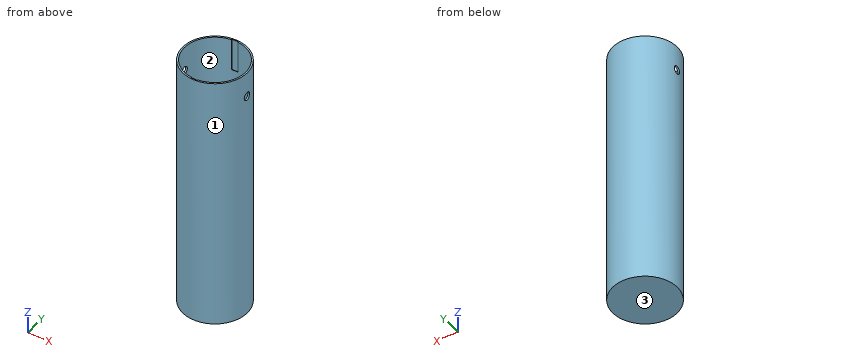
from build123d import *

# Parameters (mm, degrees)
SKETCH1_R           = 10
BOSS_EXTRUDE1_DEPTH = 80
SHELL1_T            = -0.5
SKETCH4_R           = 1.25
CUT_EXTRUDE3_DEPTH  = 84.066238629
SKETCH8_W           = 2
SKETCH8_H           = 0.25
CUT_EXTRUDE5_DEPTH  = 10


with BuildPart() as part:
    # Sketch1 → Boss-Extrude1 (new body)
    with BuildSketch(Plane.XY):
        Circle(SKETCH1_R)
    extrude(amount=BOSS_EXTRUDE1_DEPTH)

    # Shell1
    shell1_openings = [part.faces().sort_by_distance(p)[0] for p in [
        (0, 0, 80),
    ]]
    offset(amount=SHELL1_T, openings=shell1_openings, kind=Kind.INTERSECTION)

    # Sketch4 → Cut-Extrude3 (cut, through all)
    with BuildSketch(Plane(origin=(10, 0, 0), x_dir=(0, 0, -1), z_dir=(1, 0, 0))):
        with Locations((-72.25, 0)):
            Circle(SKETCH4_R)
    extrude(amount=-CUT_EXTRUDE3_DEPTH, mode=Mode.SUBTRACT)

    # Sketch8 → Cut-Extrude5 (cut)
    with BuildSketch(Plane.XY.offset(80)):
        with Locations((0, -9.5)):
            Rectangle(SKETCH8_W, SKETCH8_H)
        with Locations((0, 9.5)):
            Rectangle(SKETCH8_W, SKETCH8_H)
    extrude(amount=-CUT_EXTRUDE5_DEPTH, mode=Mode.SUBTRACT)


solid = part.part
CAD build for the part. Positions are in the model's coordinates, mm. Face numbers are marked on the shaded views. Give positions to 0.01 mm unless a question says otherwise; leave off trailing zeros. Loops run counter-clockwise (first coordinate to the right, second up) from the corner with the lowest first, then second, coordinate; pieces in that order, holes last. Notation, with made-up numbers: M 86.5,56 L 120.5,56 A27 cw 120.5,92 Z; hole C -7,22 d5. An arc over 180 degrees is marked long. Write each question's results on one line, items separated by ' | '.
Q1. Band-saw the part on D-D on y = 6. Write the cut outline in (x, z).
Geometry check:
outline: M -8,0 L 8,0 L 8,80 L 7.37,80 L 7.37,0.5 L -7.37,0.5 L -7.37,80 L -8,80 Z
Q2. Band-saw the part on B-B on x = 0. Write the cut outline in (y, z) (3 decimals).
Geometry check:
outline: M -10,0 L 10,0 L 10,80 L 9.625,80 L 9.625,70 L 9.5,70 L 9.5,0.5 L -9.5,0.5 L -9.5,70 L -9.625,70 L -9.625,80 L -10,80 Z
Q3. Band-saw the part on C-C on z = 72.25. Write the cut outline in (x, y) (3 decimals), and give its area (3 significant figures).
Geometry check:
outline: M -9.922,-1.25 A10 ccw 9.922,-1.25 L 9.417,-1.25 A9.5 cw 1,-9.447 L 1,-9.625 L -1,-9.625 L -1,-9.447 A9.5 cw -9.417,-1.25 Z; M -9.922,1.25 L -9.417,1.25 A9.5 cw -1,9.447 L -1,9.625 L 1,9.625 L 1,9.447 A9.5 cw 9.417,1.25 L 9.922,1.25 A10 ccw Z | area: 27.6 mm²
Q4. Mould opens along X. For the marked faces 1, 2 and 3 say: pulls with the +X half, pulls with the -X half, needs draft (parallel to the pull), parting line crosses it, or undercut.
Geometry check:
face 1: parting line crosses it | face 2: undercut | face 3: needs draft
Q5. Band-saw the part on A-A on y = 0. Write the cut outline in (x, z).
Geometry check:
outline: M -10,0 L 10,0 L 10,71 L 9.5,71 L 9.5,0.5 L -9.5,0.5 L -9.5,71 L -10,71 Z; M -10,73.5 L -9.5,73.5 L -9.5,80 L -10,80 Z; M 9.5,73.5 L 10,73.5 L 10,80 L 9.5,80 Z
Q6. Probe probe 1 along Z at (x, y) = (9.6, 0); probe 2 along Y at (x, z) = (0, 30); probe 3 along X at (y, z) = (0.5, 50.5). List the from-to ranges inside material, lowest first.
Geometry check:
probe 1: z = 0 to 71, 73.5 to 80 | probe 2: y = -10 to -9.5, 9.5 to 10 | probe 3: x = -9.99 to -9.49, 9.49 to 9.99
Q7. Flat gauge pins, fed straight in: P1, Ø10, axis at x = 4.5, z = 39, coming from the +Y side; P2, Ø9.5, axis at x = -1.5, y = 4, coming from the +Z side; P3, Ø2, axis at y = 0, z = 72.25, coming from the -X side; P4, Ø1.5, axis at x = 4, z = 67, coming from the -Y side. Where does each tip first touch, or does it go through?
Geometry check:
P1: stops at y = 10 | P2: stops at z = 0.5 | P3: passes through | P4: stops at y = -9.46
